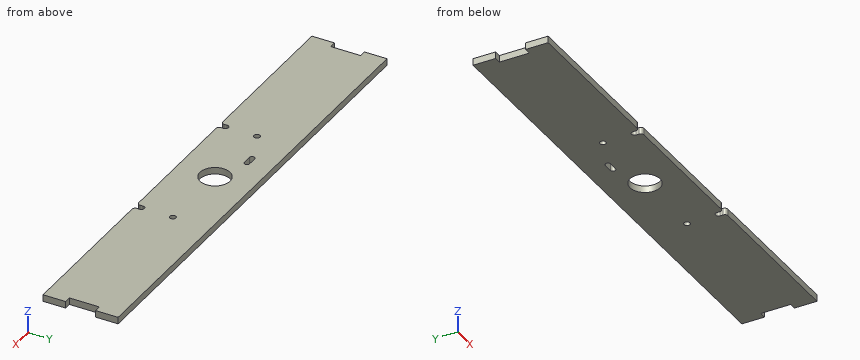
```python
from build123d import *

# Parameters (mm, degrees)
SKETCH1_W                        = 406.4
SKETCH1_H                        = 63.5
BOSS_EXTRUDE1_DEPTH              = 5.715
SKETCH2_R                        = 12.7
SEED_HOLE_DEPTH                  = 6.715
SEED_HOLE_DEPTH_BACK             = 1
SKETCH3_R                        = 2.54
LED_MOUNT_DEPTH                  = 6.715
IR_SENSOR_WIRE_KEEPER_DEPTH      = 1
IR_SENSOR_WIRE_KEEPER_DEPTH_BACK = 6.715
FILLET1_R                        = 2.54
SEED_SWITCH_MOUNT_DEPTH          = 6.715
SKETCH6_W                        = 5.715
SKETCH6_H                        = 25.4
CUT_EXTRUDE6_DEPTH               = 6.715


with BuildPart() as part:
    # Sketch1 → Boss-Extrude1 (new body)
    with BuildSketch(Plane.XY):
        Rectangle(SKETCH1_W, SKETCH1_H)
    extrude(amount=BOSS_EXTRUDE1_DEPTH)

    # Sketch2 → Seed Hole (cut, two sides)
    with BuildSketch(Plane.XY) as seed_hole_sk:
        Circle(SKETCH2_R)
    extrude(amount=SEED_HOLE_DEPTH, mode=Mode.SUBTRACT)
    extrude(seed_hole_sk.sketch, amount=-SEED_HOLE_DEPTH_BACK, mode=Mode.SUBTRACT)

    # Sketch3 → LED Mount (cut, through all)
    with BuildSketch(Plane.XY):
        with Locations((-63.5, 0)):
            Circle(SKETCH3_R)
        with Locations((63.5, 0)):
            Circle(SKETCH3_R)
    extrude(amount=LED_MOUNT_DEPTH, mode=Mode.SUBTRACT)

    # Sketch4 → IR Sensor Wire Keeper (cut, two sides)
    with BuildSketch(Plane.XY.offset(5.715)) as ir_sensor_wire_keeper_sk:
        with BuildLine():
            Line((-60.96, -26.67), (-60.96, -36.83))
            ThreePointArc((-60.96, -36.83), (-63.5, -39.37), (-66.04, -36.83))
            Line((-66.04, -36.83), (-66.04, -26.67))
            ThreePointArc((-66.04, -26.67), (-63.5, -24.13), (-60.96, -26.67))
        make_face()
        with BuildLine():
            Line((66.04, -26.67), (66.04, -36.83))
            ThreePointArc((66.04, -36.83), (63.5, -39.37), (60.96, -36.83))
            Line((60.96, -36.83), (60.96, -26.67))
            ThreePointArc((60.96, -26.67), (63.5, -24.13), (66.04, -26.67))
        make_face()
    extrude(amount=IR_SENSOR_WIRE_KEEPER_DEPTH, mode=Mode.SUBTRACT)
    extrude(ir_sensor_wire_keeper_sk.sketch, amount=-IR_SENSOR_WIRE_KEEPER_DEPTH_BACK, mode=Mode.SUBTRACT)

    # Fillet1
    fillet1_edges = [part.edges().sort_by_distance(p)[0] for p in [
        (-60.96, -31.75, 2.8575),
        (-66.04, -31.75, 2.8575),
        (66.04, -31.75, 2.8575),
        (60.96, -31.75, 2.8575),
    ]]
    fillet(fillet1_edges, radius=FILLET1_R)

    # Sketch5 → Seed Switch Mount (cut, through all)
    with BuildSketch(Plane.XY.offset(5.715)):
        with BuildLine():
            Line((-35.56, 13.6525), (-27.94, 13.6525))
            ThreePointArc((-27.94, 13.6525), (-25.7175, 11.43), (-27.94, 9.2075))
            Line((-27.94, 9.2075), (-35.56, 9.2075))
            ThreePointArc((-35.56, 9.2075), (-37.7825, 11.43), (-35.56, 13.6525))
        make_face()
    extrude(amount=-SEED_SWITCH_MOUNT_DEPTH, mode=Mode.SUBTRACT)

    # Sketch6 → Cut-Extrude6 (cut, through all)
    with BuildSketch(Plane.XY.offset(5.715)):
        with Locations((-200.3425, 0)):
            Rectangle(SKETCH6_W, SKETCH6_H)
    cut_extrude6 = extrude(amount=-CUT_EXTRUDE6_DEPTH, mode=Mode.SUBTRACT)

    # Mirror1: Cut-Extrude6 across plane
    add(cut_extrude6.mirror(Plane(origin=(0, 0, 0), x_dir=(0, 0, 1), z_dir=(1, 0, 0))), mode=Mode.SUBTRACT)


solid = part.part
```
Here's how the part is built. I have some questions about the finished solid (model axes, mm). Coordinates: 2 decimals unless noted, no trailing zeros. Order: outer loops, then holes, each group sorted by start corner. A loop starts at its lowest first (then second) coordinate and runs counter-clockwise, first axis right, second up.
Item 1: If we section it at A-A, the plane x = 0: List the corners of the cut face in (y, z) for me (3 decimals), then the cut area to 3 significant figures.
Response values:
outline: (-31.75, 0) - (-12.7, 0) - (-12.7, 5.715) - (-31.75, 5.715) - close; (12.7, 0) - (31.75, 0) - (31.75, 5.715) - (12.7, 5.715) - close
area: 218 mm2
Item 2: I need wall thicknesses on probe 1 along X at (y, z) = (0, 4.2) (3 decimals); probe 2 along Y at (x, z) = (-29, 5.3); probe 3 along Y at (x, z) = (63.5, 4.4). Which ranges of each line are inside material? Lowest first, please.
Response values:
probe 1: x = -197.485 to -66.04, -60.96 to -12.7, 12.7 to 60.96, 66.04 to 197.485
probe 2: y = -31.75 to 9.21, 13.65 to 31.75
probe 3: y = -24.13 to -2.54, 2.54 to 31.75
Item 3: If we section it at B-B, the plane z = 4.2: Give the number of separate pieces and of enclosed holes in the cut face, then the cut area to 3 significant figures.
Response values:
separate pieces: 1
enclosed holes: 4
area: 24,800 mm2
Item 4: I'm going to push flat-ended pins straight in: pin 1 Ø6.5 at (x, y) = (-63.5, 0) entering from -Z; pin 2 Ø1 at (y, z) = (-4.5, 1) entering from +X (3 decimals); pin 3 Ø2 at (y, z) = (4, 4.5) entering from -X (3 decimals). Where does each tip first touch, or does it pass through?
Response values:
pin 1: stops at z = 0
pin 2: stops at x = 197.485
pin 3: stops at x = -197.485
